Work out the finished part from the listing and answer in its coordinate system (mm). Face numbers are marked on the shaded views. A direction names the side the tool comes from. Round coordinates to 2 decimals unless told otherwise and drop trailing zeros. Loops run counter-clockwise (first coordinate to the right, second up) from the corner with the lowest first, then second, coordinate; pieces in that order, holes last.
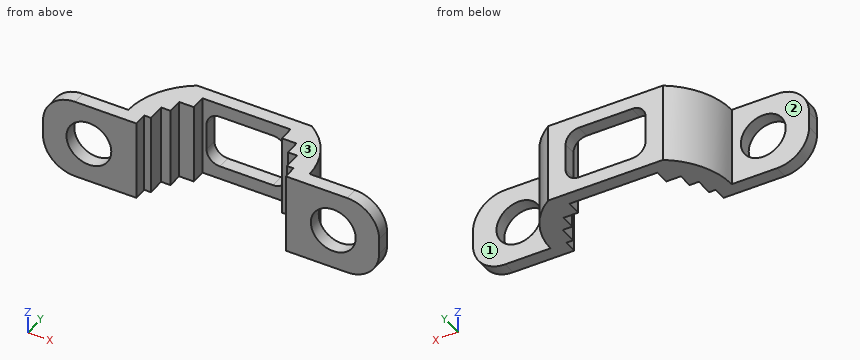
from build123d import *

# Parameters (mm, degrees)
EXTRUDE_THIN1_DEPTH  = 15
SKETCH2_R            = 8.4
CUT_EXTRUDE1_DEPTH   = 69.574794932
FILLET1_R            = 12
FILLET1_OF_MIRROR1_R = 12
SKETCH3_W            = 30
SKETCH3_H            = 20
CUT_EXTRUDE2_DEPTH   = 71.377571001
BOSS_EXTRUDE1_DEPTH  = 30
FILLET2_R            = 5


with BuildPart() as part:
    # Sketch1 → Extrude-Thin1 (new, symmetric)
    with BuildSketch(Plane.XY):
        Polygon((-63, 4.5), (-28, 4.5), (-28, 9.5), (-25.5, 9.5), (-25.5, 16), (-22, 16), (-22, 21.5), (-16.5, 21.5), (-16.5, 27.05), (0, 27.05), (0, 32.05), (-21.5, 32.05), (-21.5, 26.5), (-27, 26.5), (-27, 21), (-30.5, 21), (-30.5, 14.5), (-33, 14.5), (-33, 9.5), (-63, 9.5), align=None)
    extrude_thin1 = extrude(amount=EXTRUDE_THIN1_DEPTH, both=True)

    # Sketch2 → Cut-Extrude1 (cut, through all)
    with BuildSketch(Plane(origin=(0, 9.5, 0), x_dir=(1, 0, 0), z_dir=(0, 1, 0))):
        with Locations(Location((-45.8, 0, 0), (0, 0, 270))):
            Circle(SKETCH2_R)
    cut_extrude1 = extrude(amount=-CUT_EXTRUDE1_DEPTH, mode=Mode.SUBTRACT)

    # Fillet1
    fillet1_edges = [part.edges().sort_by_distance(p)[0] for p in [
        (-63, 7, -15),
        (-63, 7, 15),
    ]]
    fillet(fillet1_edges, radius=FILLET1_R)

    # Mirror1: Extrude-Thin1, Cut-Extrude1 across plane
    add(extrude_thin1.mirror(Plane(origin=(0, 32.05, 15), x_dir=(0, 0, 1), z_dir=(1, 0, 0))))
    add(cut_extrude1.mirror(Plane(origin=(0, 32.05, 15), x_dir=(0, 0, 1), z_dir=(1, 0, 0))), mode=Mode.SUBTRACT)

    # Fillet1 of Mirror1
    fillet1_of_mirror1_edges = [part.edges().sort_by_distance(p)[0] for p in [
        (63, 7, -15),
        (63, 7, 15),
    ]]
    fillet(fillet1_of_mirror1_edges, radius=FILLET1_OF_MIRROR1_R)

    # Sketch3 → Cut-Extrude2 (cut, through all)
    with BuildSketch(Plane(origin=(0, 32.05, 0), x_dir=(1, 0, 0), z_dir=(0, 1, 0))):
        Rectangle(SKETCH3_W, SKETCH3_H)
    extrude(amount=-CUT_EXTRUDE2_DEPTH, mode=Mode.SUBTRACT)

    # Sketch4 → Boss-Extrude1 (add)
    with BuildSketch(Plane.XY.offset(15)):
        with BuildLine():
            Line((-21.5, 26.5), (-21.5, 32.05))
            ThreePointArc((-21.5, 32.05), (-30.55647166, 22.330693825), (-34, 9.5))
            Line((-34, 9.5), (-33, 9.5))
            Line((-33, 9.5), (-33, 14.5))
            Line((-33, 14.5), (-30.5, 14.5))
            Line((-30.5, 14.5), (-30.5, 21))
            Line((-30.5, 21), (-27, 21))
            Line((-27, 21), (-27, 26.5))
            Line((-27, 26.5), (-21.5, 26.5))
        make_face()
    boss_extrude1 = extrude(amount=-BOSS_EXTRUDE1_DEPTH)

    # Mirror2: Boss-Extrude1 across plane
    add(boss_extrude1.mirror(Plane(origin=(0, 0, 0), x_dir=(0, 0, 1), z_dir=(1, 0, 0))))

    # Fillet2
    fillet2_edges = [part.edges().sort_by_distance(p)[0] for p in [
        (-15, 29.55, 10),
        (-15, 29.55, -10),
        (15, 29.55, -10),
        (15, 29.55, 10),
    ]]
    fillet(fillet2_edges, radius=FILLET2_R)


solid = part.part
Item 1: Section A-A, the plane x = -13 is taken. Give the vertices of the cut face in (y, z).
Item 2: Section B-B, the plane y = 12 is taken. Give the vertices of the cut face in (x, z).
Item 3: Each of these flat-tipped pins is pushed along its axis until it touches: P1, Ø6, axis at y = 23, z = -1.5, coming from the +X side; P2, Ø1.5, axis at y = 28.5, z = 0.5, coming from the -X side; P3, Ø3, axis at x = -25, z = -10, coming from the +Y side; P4, Ø10, axis at x = -39.5, y = 15, coming from the -Z side. Where does it stop, or does it pass through?
Item 4: Straight lines are drawn through the part: line 1 (X direction, y = 6.65, z = 0); line 2 (Z direction, x = 45.8, y = 7.6); line 3 (Y direction, x = -15.5, z = 3). For each, find the intervals that lie inside material, in ascending order.
Item 5: Section C-C, the plane z = 0 is taken. State how many separate pieces and enclosed holes the cut face has, plus the area to 3 significant figures.
Item 6: For the marked faces 1, 2 and 3, determine the directions among +Z, -Z, +X, -X, +Y, -Y from which every point of the face is accessible in a straight line to the end or side of a thin tool.
Answer below:
1. outline: (27.05, -15) - (32.05, -15) - (32.05, -9) - (27.05, -9) - close; (27.05, 9) - (32.05, 9) - (32.05, 15) - (27.05, 15) - close
2. outline: (-33.84, -15) - (-25.5, -15) - (-25.5, 15) - (-33.84, 15) - close; (25.5, -15) - (33.84, -15) - (33.84, 15) - (25.5, 15) - close
3. P1: stops at x = 31.71
3. P2: stops at x = -26.62
3. P3: stops at y = 30.62
3. P4: passes through
4. line 1: x = -63 to -54.2, -37.4 to -28, 28 to 37.4, 54.2 to 63
4. line 2: z = -15 to -8.4, 8.4 to 15
4. line 3: y = 27.05 to 32.05
5. separate pieces: 4
5. enclosed holes: 0
5. area: 639 mm2
6. face 1: +Z, -Z, +X, +Y
6. face 2: +Z, -Z, -X, +Y
6. face 3: +Z, +X, -X, +Y, -Y
